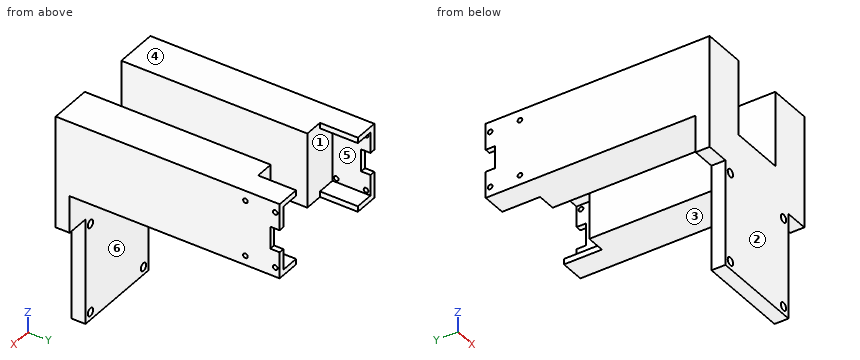
```python
from build123d import *

# Parameters (mm, degrees)
BOSS_EXTRUDE1_START = -34.5
SKETCH2_W           = 34.4
SKETCH2_H           = 20.4
SKETCH2_R           = 1.25
BOSS_EXTRUDE1_DEPTH = 3
SKETCH1_W           = 13
SKETCH1_H           = 3
BOSS_EXTRUDE2_DEPTH = 20.4
SKETCH1_3_W         = 20
SKETCH1_3_H         = 34.4
SKETCH1_3_W_2       = 10
SKETCH1_3_H_2       = 3
SKETCH1_3_W_3       = 3
BOSS_EXTRUDE3_DEPTH = 3
SKETCH1_4_W         = 3
SKETCH1_4_H         = 34.4
SKETCH1_4_W_2       = 10
SKETCH1_4_H_2       = 3
SKETCH1_4_W_3       = 20
BOSS_EXTRUDE4_DEPTH = 100
SKETCH4_W           = 12
SKETCH4_H           = 10
CUT_EXTRUDE1_DEPTH  = 132
SKETCH7_W           = 50
SKETCH7_H           = 57
SKETCH7_R           = 2.125
BOSS_EXTRUDE5_DEPTH = 7.5


with BuildPart() as part:
    # Sketch2 → Boss-Extrude1 (new body)
    with BuildSketch(Plane(origin=(0, 0, 0), x_dir=(0, 0, -1), z_dir=(1, 0, 0)).offset(BOSS_EXTRUDE1_START)):
        with Locations((0, 10.2)):
            Rectangle(SKETCH2_W, SKETCH2_H)
        with Locations((-14.8, 18)):
            Circle(SKETCH2_R, mode=Mode.SUBTRACT)
        with Locations(Location((-14.8, 2, 0), (0, 0, 180))):
            Circle(SKETCH2_R, mode=Mode.SUBTRACT)
        with Locations((15.2, 2)):
            Circle(SKETCH2_R, mode=Mode.SUBTRACT)
        with Locations(Location((15.2, 18, 0), (0, 0, 180))):
            Circle(SKETCH2_R, mode=Mode.SUBTRACT)
    extrude(amount=-BOSS_EXTRUDE1_DEPTH)

    # Sketch1 → Boss-Extrude2 (add)
    with BuildSketch(Plane(origin=(0, 0, 0), x_dir=(1, 0, 0), z_dir=(0, 1, 0))):
        with Locations((-31, -18.7)):
            Rectangle(SKETCH1_W, SKETCH1_H)
        with Locations((-31, 18.7)):
            Rectangle(SKETCH1_W, SKETCH1_H)
    extrude(amount=BOSS_EXTRUDE2_DEPTH)

    # Sketch1<3> → Boss-Extrude3 (add)
    with BuildSketch(Plane(origin=(0, 0, 0), x_dir=(1, 0, 0), z_dir=(0, 1, 0))):
        with Locations((-24.5, 0)):
            Rectangle(SKETCH1_3_W, SKETCH1_3_H)
        with Locations((-19.5, -18.7)):
            Rectangle(SKETCH1_3_W_2, SKETCH1_3_H_2)
        Polygon((-24.5, -20.2), (-24.5, -17.2), (-34.5, -17.2), (-37.5, -17.2), (-37.5, -20.2), align=None)
        with Locations((-36, 0)):
            Rectangle(SKETCH1_3_W_3, SKETCH1_3_H)
        Polygon((-34.5, 17.2), (-24.5, 17.2), (-24.5, 20.2), (-37.5, 20.2), (-37.5, 17.2), align=None)
        with Locations((-19.5, 18.7)):
            Rectangle(SKETCH1_3_W_2, SKETCH1_3_H_2)
    extrude(amount=-BOSS_EXTRUDE3_DEPTH)

    # Sketch1<4> → Boss-Extrude4 (add)
    with BuildSketch(Plane(origin=(0, 0, 0), x_dir=(1, 0, 0), z_dir=(0, 1, 0))):
        with Locations((-36, 0)):
            Rectangle(SKETCH1_4_W, SKETCH1_4_H)
        Polygon((-24.5, -20.2), (-24.5, -17.2), (-34.5, -17.2), (-37.5, -17.2), (-37.5, -20.2), align=None)
        with Locations((-19.5, -18.7)):
            Rectangle(SKETCH1_4_W_2, SKETCH1_4_H_2)
        with Locations((-24.5, 0)):
            Rectangle(SKETCH1_4_W_3, SKETCH1_4_H)
        Polygon((-34.5, 17.2), (-24.5, 17.2), (-24.5, 20.2), (-37.5, 20.2), (-37.5, 17.2), align=None)
        with Locations((-19.5, 18.7)):
            Rectangle(SKETCH1_4_W_2, SKETCH1_4_H_2)
    extrude(amount=-BOSS_EXTRUDE4_DEPTH)

    # Sketch4 → Cut-Extrude1 (cut)
    with BuildSketch(Plane(origin=(-34.5, 0, 0), x_dir=(0, 0, -1), z_dir=(1, 0, 0))):
        with Locations((0, 20.4)):
            Rectangle(SKETCH4_W, SKETCH4_H)
    extrude(amount=-CUT_EXTRUDE1_DEPTH, mode=Mode.SUBTRACT)


with BuildPart() as body_2:
    # Mirror6: mirrored copy
    add(part.part.mirror(Plane(origin=(0, 0, 0), x_dir=(0, 0, 1), z_dir=(1, 0, 0))))


with BuildPart() as part_1:
    add(part.part)

    add(body_2.part)  # Boss-Extrude5 merges body 2
    # Sketch7 → Boss-Extrude5 (add)
    # profile 1 of 2: a face of its own
    with BuildSketch(Plane.XZ.offset(100)):
        Polygon((-14.5, -20.2), (14.5, -20.2), (37.5, -20.2), (37.5, -40.2), (-37.5, -40.2), (-37.5, -20.2), align=None)
    # profile 2 of 2: a face of its own
    with BuildSketch(Plane.XZ.offset(100)):
        with Locations((0, -68.7)):
            Rectangle(SKETCH7_W, SKETCH7_H)
        with Locations(Location((-21.035, -92.99, 0), (0, 0, 270))):
            Circle(SKETCH7_R, mode=Mode.SUBTRACT)
        with Locations(Location((-21.035, -44.95, 0), (0, 0, 270))):
            Circle(SKETCH7_R, mode=Mode.SUBTRACT)
        with Locations(Location((21.035, -92.99, 0), (0, 0, 270))):
            Circle(SKETCH7_R, mode=Mode.SUBTRACT)
        with Locations(Location((21.035, -44.95, 0), (0, 0, 270))):
            Circle(SKETCH7_R, mode=Mode.SUBTRACT)
    extrude(amount=-BOSS_EXTRUDE5_DEPTH)


solid = part_1.part
```
Design review of the part built by this model. Coordinates are the model's own, in mm. Face numbers are marked on the shaded views. A direction names the side the tool comes from. Coordinates: 2 decimals unless noted, no trailing zeros. Order: outer loops, then holes, each group sorted by start corner. A loop starts at its lowest first (then second) coordinate and runs counter-clockwise, first axis right, second up.
1) Wall thickness on line 1 along X through (y, z) = (-98, -92.99); line 2 along X through (y, z) = (-36.5, 2); line 3 along Y through (x, z) = (-10.5, -23): over which ranges is each line inside the solid? List them lowest first.
2) Take a section at B-B, the plane y = -14.5. Give the boundary of the cut face in (x, z), and give its area (3 significant figures).
3) Clearance check with flat-ended pins moving along their axes: pin 1 (2 mm diameter, centred on x = -13, z = -66, fed in from +Y); pin 2 (8 mm diameter, centred on x = -0.5, y = -98, fed in from +Z); pin 3 (2 mm diameter, centred on y = 18, z = 14.8, fed in from -X) (3 decimals); pin 4 (10 mm diameter, centred on x = -22.5, z = 8.5, fed in from +Y). State where each tip first meets the part, or that it passes through.
4) Take a section at D-D, the plane x = -26.5. Give the boundary of the cut face in (y, z).
5) Take a section at A-A, the plane z = -44.95. Give the boundary of the cut face in (x, y).
6) For the marked faces 4, 5 and 6, list the 3-axis set-ups (+Z, -Z, +X, -X, +Y, -Y) from which the entire face can be reached by the end or side of a thin tool; tool diameter is ignored.
7) Take a section at C-C, the plane z = -10. Give the boundary of the cut face in (x, y).
8) Mouldability with a two-part tool opening along Z and no side actions: class the marked faces 1, 2 and 3 as +Z half, -Z half, draft (parallel to the pull), parting line (faces both ways), or undercut.
Returned:
1. line 1: x = -25 to -23.16, -18.91 to 18.91, 23.16 to 25
1. line 2: x = -37.5 to -14.5, 14.5 to 37.5
1. line 3: y = -100 to -92.5
2. outline: (-37.5, -20.2) - (-14.5, -20.2) - (-14.5, 20.2) - (-37.5, 20.2) - close; (14.5, -20.2) - (37.5, -20.2) - (37.5, 20.2) - (14.5, 20.2) - close
2. area: 1,860 mm2
3. pin 1: stops at y = -92.5
3. pin 2: stops at z = -20.2
3. pin 3: passes through
3. pin 4: stops at y = 0
4. outline: (-100, -40.2) - (-92.5, -40.2) - (-92.5, -20.2) - (20.4, -20.2) - (20.4, -17.2) - (0, -17.2) - (0, 17.2) - (20.4, 17.2) - (20.4, 20.2) - (-100, 20.2) - close
5. outline: (-25, -100) - (-23.16, -100) - (-23.16, -92.5) - (-25, -92.5) - close; (-18.91, -100) - (18.91, -100) - (18.91, -92.5) - (-18.91, -92.5) - close; (23.16, -100) - (25, -100) - (25, -92.5) - (23.16, -92.5) - close
6. face 4: +Z, +X, -X, +Y, -Y
6. face 5: +Y
6. face 6: -Z, +X, -X, +Y
7. outline: (-37.5, -100) - (-14.5, -100) - (-14.5, 0) - (-34.5, 0) - (-34.5, 20.4) - (-37.5, 20.4) - close; (14.5, -100) - (37.5, -100) - (37.5, 20.4) - (34.5, 20.4) - (34.5, 0) - (14.5, 0) - close
8. face 1: undercut
8. face 2: draft
8. face 3: -Z half
